For this review, take the finished solid that the model builds, in its own axes (mm). A direction names the side the tool comes from. Give positions to 0.01 mm unless a question says otherwise; leave off trailing zeros. Write each loop counter-clockwise with the first axis right and the second up, starting at its lowest first coordinate (ties: lowest second). Pieces come first, ordered by that corner, then holes.
1) We need section C-C on y = 1.4. Give the number of separate pieces and of enclosed holes in the cut face, and give its area (3 significant figures).
2) For P1, Ø0.9, axis at y = 2, z = -8, coming from the -X side, flat-tipped, find the tip position at first contact; note if it passes through.
3) We need section A-A on z = -1.75. Give the boundary of the cut face in (x, y), and give its area (3 significant figures).
4) Draft analysis for pull direction X (two halves, no side actions). For faces 4 (the face through (0.85, 1.52, -4.14)), 5 (the face through (15.42, 1.52, -17.26)), 6 (the face through (15, 3, -10)), 7 (the face through (12.465, 1.521, -17.307)), state which applies: pulls with the +X half, pulls with the -X half, needs draft (parallel to the pull), parting line crosses it, or undercut.
5) We need section B-B on x = 2. Give the boundary of the cut face in (y, z).
6) Wall thickness on line 1 along X through (y, z) = (1.2, -15.75); line 2 along X through (y, z) = (1.35, -2.25); line 3 along X through (y, z) = (1.9, -10.25): over which ranges is each line inside the solid? List them lowest first.
7) We need section D-D on z = -10.5. Give the boundary of the cut face in (x, y), and give its area (3 significant figures).
8) Machinability: for faces 1 (the face through (2.974, 1, -9)), 2 (the face through (3.17, 1.52, -3.32)), 3 (the face through (29.795, 1.479, -4.253)), which of the approach directions +Z, -Z, +X, -X, +Y, -Y give a long, thin tool a straight path to every point of the face, cutting with its end or side? Answer none if there is none.
from build123d import *

# Parameters (mm, degrees)
SKETCH1_W           = 30.65
SKETCH1_H           = 19.11
BOSS_EXTRUDE1_DEPTH = 3
SKETCH4_W           = 3.107341839
SKETCH4_H           = 7.887877928
CUT_EXTRUDE1_DEPTH  = 37.243821542
FILLET5_R           = 3
SKETCH5_W           = 2.973903927
SKETCH5_H           = 7.883841559
CUT_EXTRUDE2_DEPTH  = 37.243821542
FILLET6_R           = 3
FILLET7_R           = 3
SKETCH6_R           = 1.147476531
SKETCH6_R_2         = 1.171812298
SKETCH6_R_3         = 1.204786214
SKETCH6_R_4         = 1.179845326
CUT_EXTRUDE3_DEPTH  = 37.243821542
SKETCH7_R           = 0.553427196
SKETCH7_R_2         = 0.52616078
SKETCH7_R_3         = 0.51162232
SKETCH7_R_4         = 0.570497963
SKETCH7_R_5         = 0.574861319
SKETCH7_R_6         = 0.542267602
SKETCH7_R_7         = 0.579469216
SKETCH7_R_8         = 0.558015666
SKETCH7_R_9         = 0.586205708
CUT_EXTRUDE4_DEPTH  = 37.243821542


with BuildPart() as part:
    # Sketch1 → Boss-Extrude1 (new body)
    with BuildSketch(Plane(origin=(0, 0, 0), x_dir=(1, 0, 0), z_dir=(0, 1, 0))):
        with Locations((15.325, 9.555)):
            Rectangle(SKETCH1_W, SKETCH1_H)
    extrude(amount=BOSS_EXTRUDE1_DEPTH)

    # Sketch4 → Cut-Extrude1 (cut, through all)
    with BuildSketch(Plane(origin=(0, 3, 0), x_dir=(1, 0, 0), z_dir=(0, 1, 0))):
        with Locations((29.096329081, 9.099362482)):
            Rectangle(SKETCH4_W, SKETCH4_H)
    extrude(amount=-CUT_EXTRUDE1_DEPTH, mode=Mode.SUBTRACT)

    # Fillet5
    fillet5_edges = [part.edges().sort_by_distance(p)[0] for p in [
        (30.65, 1.5, -13.043301446),
        (30.65, 1.5, -5.155423518),
    ]]
    fillet(fillet5_edges, radius=FILLET5_R)

    # Sketch5 → Cut-Extrude2 (cut, through all)
    with BuildSketch(Plane(origin=(0, 3, 0), x_dir=(1, 0, 0), z_dir=(0, 1, 0))):
        with Locations((1.486951964, 8.991865097)):
            Rectangle(SKETCH5_W, SKETCH5_H)
    extrude(amount=-CUT_EXTRUDE2_DEPTH, mode=Mode.SUBTRACT)

    # Fillet6
    # the kernel refuses this fillet: 3 mm, written as the material it takes off along each edge
    with BuildSketch(Plane(origin=(0, 10.5, -12.933785877), x_dir=(1, 0, 0), z_dir=(0, -1, 0))) as fillet6_piece_1_section:
        with BuildLine():
            CenterArc((FILLET6_R, -FILLET6_R), FILLET6_R, 90, 90)
            Line((0, -FILLET6_R), (0, 0))
            Line((0, 0), (FILLET6_R, 0))
        make_face()
    fillet6_piece_1 = extrude(amount=18, mode=Mode.PRIVATE)
    fillet6_piece_1 = split(fillet6_piece_1, bisect_by=Plane(origin=(2.973903927, 10.5, -12.933785877), z_dir=(-1, 0, 0)), keep=Keep.TOP, mode=Mode.PRIVATE)
    add(fillet6_piece_1, mode=Mode.SUBTRACT)
    with BuildSketch(Plane(origin=(0, 10.5, -5.049944318), x_dir=(0, 0, 1), z_dir=(0, -1, 0))) as fillet6_piece_2_section:
        with BuildLine():
            CenterArc((FILLET6_R, -FILLET6_R), FILLET6_R, 90, 90)
            Line((0, -FILLET6_R), (0, 0))
            Line((0, 0), (FILLET6_R, 0))
        make_face()
    fillet6_piece_2 = extrude(amount=18, mode=Mode.PRIVATE)
    fillet6_piece_2 = split(fillet6_piece_2, bisect_by=Plane(origin=(2.973903927, 10.5, -5.049944318), z_dir=(-1, 0, 0)), keep=Keep.TOP, mode=Mode.PRIVATE)
    add(fillet6_piece_2, mode=Mode.SUBTRACT)

    # Fillet7
    # the kernel refuses this fillet: 3 mm, written as the material it takes off along each edge
    with BuildSketch(Plane(origin=(0, -7.5, -19.11), x_dir=(0, 0, 1), z_dir=(0, 1, 0)), Plane(origin=(30.65, -7.5, -19.11), x_dir=(-1, 0, 0), z_dir=(0, 1, 0))) as fillet7_piece_1:
        with BuildLine():
            CenterArc((FILLET7_R, FILLET7_R), FILLET7_R, 180, 90)
            Line((0, FILLET7_R), (-FILLET7_R * 0.02, FILLET7_R))
            Line((-FILLET7_R * 0.02, FILLET7_R), (-FILLET7_R * 0.02, -FILLET7_R * 0.02))
            Line((-FILLET7_R * 0.02, -FILLET7_R * 0.02), (FILLET7_R, -FILLET7_R * 0.02))
            Line((FILLET7_R, -FILLET7_R * 0.02), (FILLET7_R, 0))
        make_face()
    extrude(amount=18, mode=Mode.SUBTRACT)
    with BuildSketch(Plane(origin=(30.65, -7.196653113, 0), x_dir=(0, 0, -1), z_dir=(0, 1, 0))) as fillet7_piece_2:
        with BuildLine():
            CenterArc((3, 2.878661245), FILLET7_R, 180, 73.64872792)
            Line((0, 2.878661245), (-0.06, 2.878661245))
            Line((-0.06, 2.878661245), (-0.06, 0))
            Line((-0.06, 0), (0, -0.06))
            ThreePointArc((0, -0.06), (1.077711759, -0.06), (2.138531988, -0.057573225))
            Line((2.138531988, -0.057573225), (2.155423518, 0))
        make_face()
    extrude(amount=17.393306227, mode=Mode.SUBTRACT)
    with BuildSketch(Plane(origin=(0, -7.113980163, 0), x_dir=(0, 0, -1), z_dir=(0, 1, 0))) as fillet7_piece_3:
        with BuildLine():
            CenterArc((3, -2.845592065), FILLET7_R, 108.462579453, 71.537420547)
            Line((0, -2.845592065), (-0.06, -2.845592065))
            Line((-0.06, -2.845592065), (-0.06, 0))
            Line((-0.06, 0), (0, 0.06))
            ThreePointArc((0, 0.06), (1.024972159, 0.06), (2.030943204, 0.056911841))
            Line((2.030943204, 0.056911841), (2.049944318, 0))
        make_face()
    extrude(amount=17.227960325, mode=Mode.SUBTRACT)

    # Sketch6 → Cut-Extrude3 (cut, through all)
    with BuildSketch(Plane(origin=(0, 3, 0), x_dir=(1, 0, 0), z_dir=(0, 1, 0))):
        with Locations(Location((2.397675936, 2.472562033, 0), (0, 0, 270))):
            Circle(SKETCH6_R)
        with Locations(Location((2.397675936, 15.534628547, 0), (0, 0, 270))):
            Circle(SKETCH6_R_2)
        with Locations(Location((28.233356839, 15.652120685, 0), (0, 0, 270))):
            Circle(SKETCH6_R_3)
        with Locations(Location((28.283999857, 2.604300321, 0), (0, 0, 270))):
            Circle(SKETCH6_R_4)
    extrude(amount=-CUT_EXTRUDE3_DEPTH, mode=Mode.SUBTRACT)

    # Sketch7 → Cut-Extrude4 (cut, through all)
    with BuildSketch(Plane(origin=(0, 3, 0), x_dir=(1, 0, 0), z_dir=(0, 1, 0))):
        with Locations(Location((25.603735312, 17.875013179, 0), (0, 0, 270))):
            Circle(SKETCH7_R)
        with Locations(Location((23.018273663, 17.875013179, 0), (0, 0, 270))):
            Circle(SKETCH7_R_2)
        with Locations(Location((20.414641054, 17.875013179, 0), (0, 0, 270))):
            Circle(SKETCH7_R_3)
        with Locations(Location((17.832185275, 17.808085307, 0), (0, 0, 270))):
            Circle(SKETCH7_R_4)
        with Locations(Location((15.250588263, 17.808085307, 0), (0, 0, 270))):
            Circle(SKETCH7_R_5)
        with Locations(Location((12.672951441, 17.808085307, 0), (0, 0, 270))):
            Circle(SKETCH7_R_6)
        with Locations(Location((10.081016635, 17.756783748, 0), (0, 0, 270))):
            Circle(SKETCH7_R_7)
        with Locations(Location((7.479204756, 17.756783748, 0), (0, 0, 270))):
            Circle(SKETCH7_R_8)
        with Locations(Location((4.895679995, 17.710489857, 0), (0, 0, 270))):
            Circle(SKETCH7_R_9)
    extrude(amount=-CUT_EXTRUDE4_DEPTH, mode=Mode.SUBTRACT)


solid = part.part
Results list:
1. separate pieces: 1
1. enclosed holes: 13
1. area: 497 mm2
2. P1: stops at x = 2.97
3. outline: (0.12, 0) - (1.51, 0) - (1.51, 3) - (0.12, 3) - close; (3.29, 0) - (27.47, 0) - (27.47, 3) - (3.29, 3) - close; (29.1, 0) - (30.5, 0) - (30.5, 3) - (29.1, 3) - close
3. area: 80.9 mm2
4. face 4: pulls with the -X half
4. face 5: undercut
4. face 6: needs draft
4. face 7: undercut
5. outline: (0, -18.94) - (3, -18.94) - (3, -16.64) - (0, -16.64) - close; (0, -14.43) - (3, -14.43) - (3, -13.11) - (0, -13.11) - close; (0, -4.88) - (3, -4.88) - (3, -3.55) - (0, -3.55) - close; (0, -1.4) - (3, -1.4) - (3, -0.12) - (0, -0.12) - close
6. line 1: x = 0.01 to 1.25, 3.55 to 27.03, 29.43 to 30.64
6. line 2: x = 0.01 to 1.27, 3.52 to 27.16, 29.41 to 30.65
6. line 3: x = 2.97 to 27.54
7. outline: (2.97, 0) - (27.54, 0) - (27.54, 3) - (2.97, 3) - close
7. area: 73.7 mm2
8. face 1: -X, +Y, -Y
8. face 2: +Y, -Y
8. face 3: +X, +Y, -Y
